The listing builds one solid part. Answer for the finished solid, in the listing's coordinates (mm). A direction names the side the tool comes from. Round coordinates to 2 decimals unless told otherwise and drop trailing zeros. Order: outer loops, then holes, each group sorted by start corner. A loop starts at its lowest first (then second) coordinate and runs counter-clockwise, first axis right, second up. Notation, with made-up numbers: (8, 43) - (48, 43) arc R9 ccw to (48, 56) - close; hole circle Ø7 at (45.5, 46.25). An arc over 180 degrees is marked (long way). Use CSV: the item, a comma, the result in double quotes. Start each with the question number.
Item 1: Flat-ended cylindrical pins translate along their axes: P1, Ø4, axis at y = -32.5, z = -7, coming from the +X side; P2, Ø4, axis at y = -36.5, z = -12, coming from the -X side; P3, Ø4.5, axis at x = 88, y = -33.5, coming from the -Z side. Find the tip coordinate at first contact, or state that the pin passes through.
Item 2: Find section C-C, the plane y = -40.5. Give the vertices of the cut face in (x, z), plus the area to 3 significant figures.
Item 3: Straight lines are drawn through the part: line 1 along Y through (x, z) = (97, -1); line 2 along Y through (x, z) = (101.5, -13); line 3 along Z through (x, y) = (89, -34.75). For each, find the intervals that lie inside material, in ascending order. Write a range as [from, to].
Item 4: Find section A-A, the plane x = 88. Give the vertices of the cut face in (y, z).
Item 5: Find section B-B, the plane z = -8.5. Give the vertices of the cut face in (x, y), plus the area to 3 significant figures.
Item 6: For faces 4 (the flat face through (88, -30, -11)), 5 (the cylindrical face through (82.006, -32.958, -8.236)), 6 (the flat face through (89.1, -42, 5.4)), determine the directions among +Z, -Z, +X, -X, +Y, -Y from which every point of the face is accessible in a straight line to the end or side of a thin tool.
Item 7: Determine the mould class of faces 1 (the flat face through (102, -38, -14)), 2 (the flat face through (88, -33, -10.096)), 3 (the cylindrical face through (75.7, -42.99, -17.93)) for opening direction Z: +Z half, -Z half, draft (parallel to the pull), parting line (faces both ways), or undercut.
```python
from build123d import *

# Parameters (mm, degrees)
CYLINDER033_R         = 15.5
CYLINDER033_DEPTH     = 2
CYLINDER032_R         = 13.5
CYLINDER032_DEPTH     = 5
CYLINDER034_R         = 15.5
CYLINDER034_DEPTH     = 2
EXTRUDE001_DEPTH      = 7
CYLINDER031_R         = 6
CYLINDER031_DEPTH     = 14
CHAMFER005_SIZE       = 1
CHAMFER005_ROLL_ANGLE = 90


with BuildPart() as cilindro030:
    # Cylinder033 → Cylinder033 (new body)
    with BuildSketch(Plane(origin=(-1, 25, 36), x_dir=(1, 0, 0), z_dir=(0, 0, 1))):
        Circle(CYLINDER033_R)
    extrude(amount=CYLINDER033_DEPTH)


with BuildPart() as cilindro029:
    # Cylinder032 → Cylinder032 (new body)
    with BuildSketch(Plane(origin=(-1, 25, 31), x_dir=(1, 0, 0), z_dir=(0, 0, 1))):
        Circle(CYLINDER032_R)
    extrude(amount=CYLINDER032_DEPTH)


with BuildPart() as cilindro031:
    # Cylinder034 → Cylinder034 (new body)
    with BuildSketch(Plane(origin=(-1, 25, 30), x_dir=(1, 0, 0), z_dir=(0, 0, 1))):
        Circle(CYLINDER034_R)
    extrude(amount=CYLINDER034_DEPTH)


with BuildPart() as extrude001:
    # Sketch001 → Extrude001 (new body)
    with BuildSketch(Plane.XY):
        with BuildLine():
            Line((-2.060088, 8.599999), (2.000001, 8.599999))
            ThreePointArc((2.000001, 5.404159), (2.598634, 7.002079), (2.000001, 8.599999))
            Line((2.000001, 5.404159), (-2.060088, 5.404159))
            ThreePointArc((-2.060088, 8.599999), (-2.651924, 7.002079), (-2.060088, 5.404159))
        make_face()
    extrude(amount=EXTRUDE001_DEPTH)


with BuildPart() as extrude001_1:
    # Extrude001 placement: moved
    add(extrude001.part.moved(Location((-1, 18, 24))))


with BuildPart() as polea_motor:
    # Cylinder031 → Cylinder031 (new body)
    with BuildSketch(Plane(origin=(-1, 25, 24), x_dir=(1, 0, 0), z_dir=(0, 0, 1))):
        Circle(CYLINDER031_R)
    extrude(amount=CYLINDER031_DEPTH)

    # Cut027: cut Extrude001
    add(extrude001_1.part, mode=Mode.SUBTRACT)

    # Fusion005: union Cilindro030, Cilindro029, Cilindro031
    add(cilindro030.part)
    add(cilindro029.part)
    add(cilindro031.part)

    # Chamfer005
    chamfer005_edges = [polea_motor.edges().sort_by_distance(p)[0] for p in [
        (-14.5, 25, 32),
    ]]
    chamfer(chamfer005_edges, length=CHAMFER005_SIZE)


with BuildPart() as polea_motor_1:
    # Chamfer005 roll: moved
    add(polea_motor.part.rotate(Axis((0, 0, 0), (1, 0, 0)), CHAMFER005_ROLL_ANGLE))


with BuildPart() as polea_motor_2:
    # Chamfer005 placement: moved
    add(polea_motor_1.part.moved(Location((89, -6, -33.5))))


solid = polea_motor_2.part
```
Worked out:
1,P1,"stops at x = 94"
1,P2,"stops at x = 72.57"
1,P3,"stops at z = -14.5"
2,outline,"circle Ø27 at (88, -8.5)"
2,area,"573 mm²"
3,line 1,"y = [-44, -36]"
3,line 2,"y = [-44, -42], [-38.27, -36]"
3,line 3,"z = [-14.42, -10.1], [-6.9, -2.58]"
4,outline,"(-44, -24) - (-42, -24) - (-42, -22) - (-39, -22) - (-38, -23) - (-38, -24) - (-36, -24) - (-36, -14.5) - (-30, -14.5) - (-30, -10.1) - (-36, -10.1) - (-36, -6.9) - (-30, -6.9) - (-30, -2.5) - (-36, -2.5) - (-36, 7) - (-38, 7) - (-38, 6) - (-39, 5) - (-42, 5) - (-42, 7) - (-44, 7) - close"
5,outline,"(72.5, -44) - (103.5, -44) - (103.5, -42) - (101.5, -42) - (101.5, -39) - (102.5, -38) - (103.5, -38) - (103.5, -36) - (94, -36) - (94, -30) - (90.6, -30) - (90.6, -36) - (85.35, -36) - (85.35, -30) - (82, -30) - (82, -36) - (72.5, -36) - (72.5, -38) - (73.5, -38) - (74.5, -39) - (74.5, -42) - (72.5, -42) - close"
5,area,"273 mm²"
6,face 4,"+Z, -Z, +X, -X, +Y"
6,face 5,"+Y"
6,face 6,"none"
7,face 1,"draft"
7,face 2,"undercut"
7,face 3,"parting line"
